CAD build for the part. Positions are in the model's coordinates, mm. Face numbers are marked on the shaded views. Round coordinates to 2 decimals unless told otherwise and drop trailing zeros. Loops run counter-clockwise (first coordinate to the right, second up) from the corner with the lowest first, then second, coordinate; pieces in that order, holes last. Notation, with made-up numbers: (80.25, -4.5) -> (90.25, -4.5) arc R12 ccw to (90.25, 4.5) -> close; hole circle Ø5 at (83, 33.5). An arc over 180 degrees is marked (long way). Answer as CSV lines item,"result".
Autodesk Inventor part; units mm, degrees
ref_plane "YZ Plane" through (0, 0, 0) normal (1, 0, 0) x (0, 1, 0)
ref_plane "XZ Plane" through (0, 0, 0) normal (0, 1, 0) x (-1, 0, 0)
ref_plane "XY Plane" through (0, 0, 0) normal (0, 0, 1) x (1, 0, 0)
sketch "スケッチ1" plane through (0, 0, 0) normal (0, 0, 1) x (1, 0, 0)
  arc A0 (10, -1.7157) -> (-10, -1.7157) centre (0, -30) ccw
  line L0 (-10, -1.7157) -> (-10, 9.2843)
  line L1 (-10, 9.2843) -> (10, 9.2843)
  line L2 (10, 9.2843) -> (10, -1.7157)
  line L3 (-14, 0) -> (14, 0)
  point P0 (0, 0)
  point P1 (0, 0)
  dimension "d0" = 20
  dimension "d1" = 11
  dimension "d2" = 30
extrude "押し出し1" add sketch "スケッチ1" along normal blind 4.5
fillet "フィレット1" radius 4 4 edges at (-10, 9.2843, 2.25) (10, 9.2843, 2.25) (10, -1.7157, 2.25) (-10, -1.7157, 2.25)
sketch "スケッチ2" plane through (0, 0, 4.5) normal (0, 0, 1) x (1, 0, 0)
  circle A0 centre (-4, 5.2843) radius 1.5
  circle A1 centre (4, 5.2843) radius 1.5
  line L0 (6, 9.2843) -> (-6, 9.2843)
  point P0 (0, 0)
  dimension "d7" = 3
  dimension "d8" = 3
  dimension "d9" = 4
  dimension "d10" = 4
  dimension "d11" = 4
  dimension "d12" = 4
extrude "押し出し2" cut sketch "スケッチ2" against normal blind 7.5
equation "\"d8\" = d7"
properties part number "ruber"
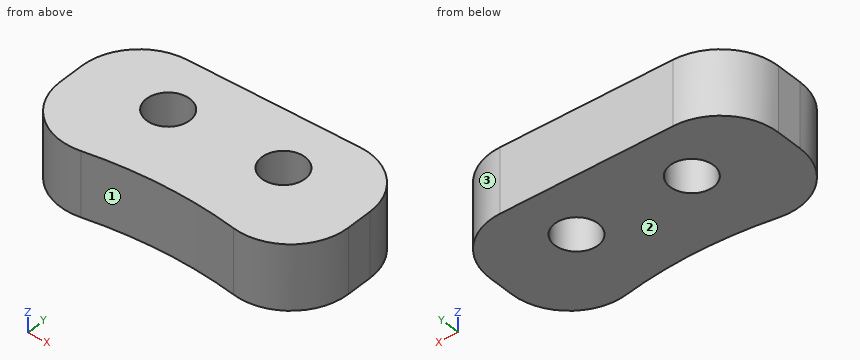
Q1. Slice it at A-A, the plane z = 0.95. Give the cut face in (x, y).
Results:
outline,"(-10, 3.47) arc R4 ccw to (-5.29, -0.47) arc R30 cw to (5.29, -0.47) arc R4 ccw to (10, 3.47) -> (10, 5.28) arc R4 ccw to (6, 9.28) -> (-6, 9.28) arc R4 ccw to (-10, 5.28) -> close; hole circle Ø3 at (-4, 5.28); hole circle Ø3 at (4, 5.28)"
Q2. Drop flat-ended pins along their axis: pin 1 Ø2.5 at (x, y) = (-4, 5.28) entering from +Z; pin 2 Ø3.5 at (x, y) = (4, 5.28) entering from -Z; pin 3 Ø2 at (y, z) = (7.5, 4) entering from +X. Give the stop position or say it passes through.
Results:
pin 1,"through"
pin 2,"z = 0"
pin 3,"x = 9.81"
Q3. Slice it at B-B, the plane x = -3.75. Give the cut face in (y, z), and give its area (3 significant figures).
Results:
outline,"(-0.24, 0) -> (3.81, 0) -> (3.81, 4.5) -> (-0.24, 4.5) -> close; (6.76, 0) -> (9.28, 0) -> (9.28, 4.5) -> (6.76, 4.5) -> close"
area,"29.5 mm2"
Q4. Two-plate mould, pull along X, no slides. Class the marked faces 1, 2 and 3: pulls with the +X half, pulls with the -X half, needs draft (parallel to the pull), parting line crosses it, or undercut.
Results:
face 1,"undercut"
face 2,"needs draft"
face 3,"pulls with the +X half"
Q5. Slice it at C-C, the plane x = 4. Give the cut face in (y, z).
Results:
outline,"(-0.27, 0) -> (3.78, 0) -> (3.78, 4.5) -> (-0.27, 4.5) -> close; (6.78, 0) -> (9.28, 0) -> (9.28, 4.5) -> (6.78, 4.5) -> close"
Q6. Slice it at D-D, the plane y = 8.5. Give the cut face in (x, z).
Results:
outline,"(-8.38, 0) -> (8.38, 0) -> (8.38, 4.5) -> (-8.38, 4.5) -> close"
Q7. Probe L1, parallel to X at y = 6.25, z = 3; L2, parallel to Y at x = -0.25, z = 2.55; L3, parallel to X at y = 4.25, z = 2.2. List the from-to ranges inside material, lowest first. Write a range as [from, to].
Results:
L1,"[-9.88, -5.15], [-2.85, 2.85], [5.15, 9.88]"
L2,"[0, 9.28]"
L3,"[-10, -5.09], [-2.91, 2.91], [5.09, 10]"
